from build123d import *

# Parameters (mm, degrees)
SKETCH1_R           = 1.6
BOSS_EXTRUDE1_DEPTH = 1


with BuildPart() as part:
    # Sketch1 → Boss-Extrude1 (new body)
    with BuildSketch(Plane.XY):
        with BuildLine():
            Line((202.085666764, -21.015048426), (202.085666764, -30.015048426))
            ThreePointArc((202.085666764, -30.015048426), (201.792773545, -30.722155207), (201.085666764, -31.015048426))
            Line((201.085666764, -31.015048426), (-26.914333236, -31.015048426))
            ThreePointArc((-26.914333236, -31.015048426), (-27.621440018, -30.722155207), (-27.914333236, -30.015048426))
            Line((-27.914333236, -30.015048426), (-27.914333236, -21.015048426))
            Line((-27.914333236, -21.015048426), (-32.914333236, -21.015048426))
            ThreePointArc((-32.914333236, -21.015048426), (-36.449867142, -19.550582332), (-37.914333236, -16.015048426))
            Line((-37.914333236, -16.015048426), (-37.914333236, 23.984951574))
            ThreePointArc((-37.914333236, 23.984951574), (-36.449867142, 27.52048548), (-32.914333236, 28.984951574))
            Line((-32.914333236, 28.984951574), (-27.914333236, 28.984951574))
            Line((-27.914333236, 28.984951574), (-27.914333236, 37.984951574))
            ThreePointArc((-27.914333236, 37.984951574), (-27.621440018, 38.692058356), (-26.914333236, 38.984951574))
            Line((-26.914333236, 38.984951574), (201.085666764, 38.984951574))
            ThreePointArc((201.085666764, 38.984951574), (201.792773545, 38.692058356), (202.085666764, 37.984951574))
            Line((202.085666764, 37.984951574), (202.085666764, 28.984951574))
            Line((202.085666764, 28.984951574), (207.085666764, 28.984951574))
            ThreePointArc((207.085666764, 28.984951574), (210.62120067, 27.52048548), (212.085666764, 23.984951574))
            Line((212.085666764, 23.984951574), (212.085666764, -16.015048426))
            ThreePointArc((212.085666764, -16.015048426), (210.62120067, -19.550582332), (207.085666764, -21.015048426))
            Line((207.085666764, -21.015048426), (202.085666764, -21.015048426))
        make_face()
        with Locations((-24.914333236, 35.984951574)):
            Circle(SKETCH1_R, mode=Mode.SUBTRACT)
        with Locations((14.085666764, 35.984951574)):
            Circle(SKETCH1_R, mode=Mode.SUBTRACT)
        with Locations((-24.914333236, -28.015048426)):
            Circle(SKETCH1_R, mode=Mode.SUBTRACT)
        with Locations((14.085666764, -28.015048426)):
            Circle(SKETCH1_R, mode=Mode.SUBTRACT)
        with Locations((21.085666764, 35.984951574)):
            Circle(SKETCH1_R, mode=Mode.SUBTRACT)
        with Locations((60.085666764, 35.984951574)):
            Circle(SKETCH1_R, mode=Mode.SUBTRACT)
        with Locations((60.085666764, -28.015048426)):
            Circle(SKETCH1_R, mode=Mode.SUBTRACT)
        with Locations((21.085666764, -28.015048426)):
            Circle(SKETCH1_R, mode=Mode.SUBTRACT)
        with Locations((67.085666764, 35.984951574)):
            Circle(SKETCH1_R, mode=Mode.SUBTRACT)
        with Locations((106.085666764, 35.984951574)):
            Circle(SKETCH1_R, mode=Mode.SUBTRACT)
        with Locations((106.085666764, -28.015048426)):
            Circle(SKETCH1_R, mode=Mode.SUBTRACT)
        with Locations((67.085666764, -28.015048426)):
            Circle(SKETCH1_R, mode=Mode.SUBTRACT)
        with Locations((113.085666764, 35.984951574)):
            Circle(SKETCH1_R, mode=Mode.SUBTRACT)
        with Locations((152.085666764, 35.984951574)):
            Circle(SKETCH1_R, mode=Mode.SUBTRACT)
        with Locations((152.085666764, -28.015048426)):
            Circle(SKETCH1_R, mode=Mode.SUBTRACT)
        with Locations((113.085666764, -28.015048426)):
            Circle(SKETCH1_R, mode=Mode.SUBTRACT)
        with Locations((159.085666764, 35.984951574)):
            Circle(SKETCH1_R, mode=Mode.SUBTRACT)
        with Locations((198.085666764, 35.984951574)):
            Circle(SKETCH1_R, mode=Mode.SUBTRACT)
        with Locations((198.085666764, -28.015048426)):
            Circle(SKETCH1_R, mode=Mode.SUBTRACT)
        with Locations((159.085666764, -28.015048426)):
            Circle(SKETCH1_R, mode=Mode.SUBTRACT)
        with Locations((-32.914333236, -16.015048426)):
            Circle(SKETCH1_R, mode=Mode.SUBTRACT)
        with Locations((-32.914333236, 23.984951574)):
            Circle(SKETCH1_R, mode=Mode.SUBTRACT)
        with Locations((207.085666764, 23.984951574)):
            Circle(SKETCH1_R, mode=Mode.SUBTRACT)
        with Locations((207.085666764, -16.015048426)):
            Circle(SKETCH1_R, mode=Mode.SUBTRACT)
    extrude(amount=BOSS_EXTRUDE1_DEPTH)


solid = part.part
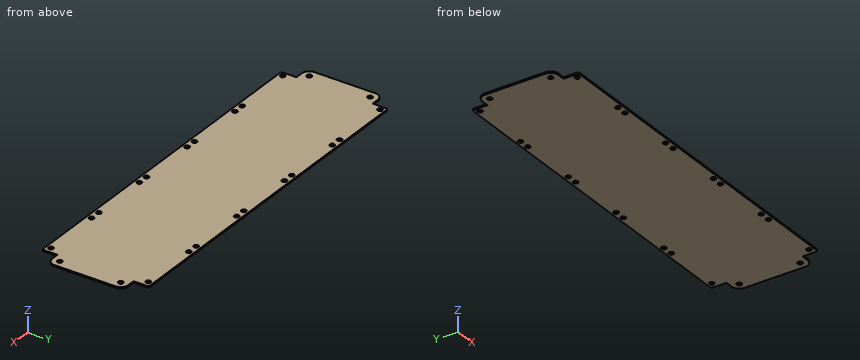
Check sheet for the modelled part. Datum: model origin and axes. Units: mm. Give positions to 0.01 mm unless a question says otherwise; leave off trailing zeros. Answer as CSV lines item,"result". Start each with the question number.
Item 1: Thickness scan on line 1 (Y direction, x = 68, z = 0.8); line 2 (X direction, y = -22.5, z = 0.9); line 3 (X direction, y = 23, z = 0.55). Record the ranges inside material, lowest first. Write a range as [from, to].
Item 2: Cross-section at A-A on z = 0.35. State how many separate pieces and enclosed holes the cut face has, plus the area to 3 significant figures.
Item 3: Gauge pin test, flat ends, axial feed: P1, Ø1.9, axis at x = 113.09, y = -28.02, coming from the -Z side; P2, Ø0.5, axis at x = -30, z = 0.5, coming from the +Y side. Record the tip position at first contact, or that the pin passes through.
Established:
1,line 1,"y = [-31.02, -29.33], [-26.7, 34.67], [37.3, 38.98]"
1,line 2,"x = [-27.91, 202.09]"
1,line 3,"x = [-37.91, -34.18], [-31.65, 205.82], [208.35, 212.09]"
2,separate pieces,"1"
2,enclosed holes,"24"
2,area,"16,900 mm^2"
3,P1,"passes through"
3,P2,"stops at y = 28.98"
